CAD build for the part. Positions are in the model's coordinates, mm. A direction names the side the tool comes from. Round coordinates to 2 decimals unless told otherwise and drop trailing zeros. Use a Markdown table: item, result. Add a question column.
(1) Wall check: L1, parallel to X at y = 8.2, z = 85.5; L2, parallel to Z at x = 17.5, y = 6.5; L3, parallel to Z at x = -13, y = 11.3. Give the ranges that are in metal, low to high.
(2) Flat gauge pins, fed straight in: P1, Ø1.5, axis at x = -23.5, z = -40, coming from the -Y side; P2, Ø18.5, axis at x = -14.5, z = 74.5, coming from the +Y side; P3, Ø10, axis at x = 15, z = -91, coming from the -Y side; P4, Ø16, axis at x = -32.5, z = 37.5, coming from the -Y side. Where does each tip first touch, or does it go through?
(3) Two-plate mould, pull along X, no slides. Class faces 4 (the face through (18, 11, -54)), 5 (the face through (-65, 8, 2)), 6 (the face through (13, 0, -2)), 7 (the face through (-34.4, 5, -5.6)): released by +X, released by -X, zero draft, split by the parting line, or undercut.
(4) Band-saw the part on A-A, the plane x = -3.5. Give the number of separate pieces and of enclosed holes in the cut face, and give its area (3 significant figures).
(5) Which spindle directions (+Z, -Z, +X, -X, +Y, -Y) get a long thin tool onto all of the face, cutting with end or side? Do faces 1 (the face through (23.114, 5.93, -60.372)), 2 (the face through (-3, 13, 92.6)), 3 (the face through (27.662, 7.528, 82.922)). Say none if no direction does.
from build123d import *

# Parameters (mm, degrees)
SKETCH1_W           = 130
SKETCH1_H           = 240
BOSS_EXTRUDE1_DEPTH = 16
SKETCH7_W           = 76.2
SKETCH7_H           = 61.2
CUT_EXTRUDE5_DEPTH  = 6
SKETCH2_R           = 2.6
CUT_EXTRUDE1_DEPTH  = 11
SKETCH8_R           = 27.1
CUT_EXTRUDE6_DEPTH  = 6
SKETCH9_R           = 2.6
CUT_EXTRUDE7_DEPTH  = 11
SKETCH5_R           = 1.55
CUT_EXTRUDE3_DEPTH  = 17
SKETCH4_R           = 10
CUT_EXTRUDE2_DEPTH  = 5
SKETCH11_R          = 10
CUT_EXTRUDE8_DEPTH  = 6
FILLET1_R           = 4
CHAMFER3_SIZE       = 2
CHAMFER1_SIZE       = 1
CHAMFER2_SIZE       = 0.5


with BuildPart() as part:
    # Sketch1 → Boss-Extrude1 (new body)
    with BuildSketch(Plane(origin=(0, 0, 0), x_dir=(1, 0, 0), z_dir=(0, 1, 0))):
        Rectangle(SKETCH1_W, SKETCH1_H)
    extrude(amount=BOSS_EXTRUDE1_DEPTH)

    # Sketch7 → Cut-Extrude5 (cut)
    with BuildSketch(Plane(origin=(0, 16, 0), x_dir=(1, 0, 0), z_dir=(0, 1, 0))):
        with Locations((-3, -62)):
            Rectangle(SKETCH7_W, SKETCH7_H)
    extrude(amount=-CUT_EXTRUDE5_DEPTH, mode=Mode.SUBTRACT)

    # Sketch2 → Cut-Extrude1 (cut, through all)
    with BuildSketch(Plane(origin=(0, 10, 0), x_dir=(1, 0, 0), z_dir=(0, 1, 0))):
        with Locations((-34, -85.5)):
            Circle(SKETCH2_R)
        with Locations((-34, -38.5)):
            Circle(SKETCH2_R)
        with Locations((28, -38.5)):
            Circle(SKETCH2_R)
        with Locations((28, -85.5)):
            Circle(SKETCH2_R)
    extrude(amount=-CUT_EXTRUDE1_DEPTH, mode=Mode.SUBTRACT)

    # Sketch8 → Cut-Extrude6 (cut)
    with BuildSketch(Plane(origin=(0, 16, 0), x_dir=(1, 0, 0), z_dir=(0, 1, 0))):
        with Locations((-13, 8)):
            Circle(SKETCH8_R)
    extrude(amount=-CUT_EXTRUDE6_DEPTH, mode=Mode.SUBTRACT)

    # Sketch9 → Cut-Extrude7 (cut, through all)
    with BuildSketch(Plane(origin=(0, 10, 0), x_dir=(1, 0, 0), z_dir=(0, 1, 0))):
        with Locations((-32, 8)):
            Circle(SKETCH9_R)
        with Locations((-3.5, 24.454482672)):
            Circle(SKETCH9_R)
        with Locations((-3.5, -8.454482672)):
            Circle(SKETCH9_R)
    extrude(amount=-CUT_EXTRUDE7_DEPTH, mode=Mode.SUBTRACT)

    # Sketch5 → Cut-Extrude3 (cut, through all)
    with BuildSketch(Plane(origin=(0, 16, 0), x_dir=(1, 0, 0), z_dir=(0, 1, 0))):
        with Locations((-18.5, 51.5)):
            Circle(SKETCH5_R)
        with Locations((-18.5, 88.5)):
            Circle(SKETCH5_R)
        with Locations((18.5, 88.5)):
            Circle(SKETCH5_R)
        with Locations((18.5, 51.5)):
            Circle(SKETCH5_R)
    extrude(amount=-CUT_EXTRUDE3_DEPTH, mode=Mode.SUBTRACT)

    # Sketch4 → Cut-Extrude2 (cut)
    with BuildSketch(Plane.XZ):
        with Locations((-34, 85.5)):
            Circle(SKETCH4_R)
        with Locations((28, 85.5)):
            Circle(SKETCH4_R)
        with Locations((28, 38.5)):
            Circle(SKETCH4_R)
        with Locations((-34, 38.5)):
            Circle(SKETCH4_R)
        with Locations((-32, -8)):
            Circle(SKETCH4_R)
        with Locations((-3.5, 8.454482672)):
            Circle(SKETCH4_R)
        with Locations((-3.5, -24.454482672)):
            Circle(SKETCH4_R)
        with Locations((-18.5, -51.5)):
            Circle(SKETCH4_R)
        with Locations((-18.5, -88.5)):
            Circle(SKETCH4_R)
        with Locations((18.5, -88.5)):
            Circle(SKETCH4_R)
        with Locations((18.5, -51.5)):
            Circle(SKETCH4_R)
    extrude(amount=-CUT_EXTRUDE2_DEPTH, mode=Mode.SUBTRACT)

    # Sketch11 → Cut-Extrude8 (cut)
    with BuildSketch(Plane.XZ.offset(-5)):
        with Locations((18.5, -88.5)):
            Circle(SKETCH11_R)
        with Locations((-18.5, -88.5)):
            Circle(SKETCH11_R)
        with Locations((-18.5, -51.5)):
            Circle(SKETCH11_R)
        with Locations((18.5, -51.5)):
            Circle(SKETCH11_R)
    extrude(amount=-CUT_EXTRUDE8_DEPTH, mode=Mode.SUBTRACT)

    # Fillet1
    fillet1_edges = [part.edges().sort_by_distance(p)[0] for p in [
        (35.1, 13, 31.4),
        (35.1, 13, 92.6),
        (-41.1, 13, 92.6),
        (-41.1, 13, 31.4),
        (-65, 8, -120),
        (65, 8, -120),
        (65, 8, 120),
        (-65, 8, 120),
    ]]
    fillet(fillet1_edges, radius=FILLET1_R)

    # Chamfer3
    chamfer3_edges = [part.edges().sort_by_distance(p)[0] for p in [
        (-65, 0, 0),
        (-65, 16, 0),
        (0, 0, -120),
        (65, 0, 0),
        (0, 0, 120),
        (63.828427125, 0, 118.828427125),
        (-63.828427125, 0, 118.828427125),
        (63.828427125, 0, -118.828427125),
        (-63.828427125, 0, -118.828427125),
        (0, 16, -120),
        (0, 16, 120),
        (65, 16, 0),
        (63.828427125, 16, 118.828427125),
        (-63.828427125, 16, 118.828427125),
        (63.828427125, 16, -118.828427125),
        (-63.828427125, 16, -118.828427125),
    ]]
    chamfer(chamfer3_edges, length=CHAMFER3_SIZE)

    # Chamfer1
    chamfer1_edges = [part.edges().sort_by_distance(p)[0] for p in [
        (-13.5, 0, -24.454482672),
        (-13.5, 0, 8.454482672),
        (-42, 0, -8),
        (-44, 0, 38.5),
        (18, 0, 38.5),
        (18, 0, 85.5),
        (8.5, 0, -88.5),
        (8.5, 0, -51.5),
        (-44, 0, 85.5),
        (35.1, 16, 62),
        (-3, 16, 92.6),
        (-41.1, 16, 62),
        (-3, 16, 31.4),
        (33.928427125, 16, 32.571572875),
        (33.928427125, 16, 91.428427125),
        (-39.928427125, 16, 91.428427125),
        (-39.928427125, 16, 32.571572875),
        (-40.1, 16, -8),
        (-28.5, 0, -88.5),
        (-28.5, 0, -51.5),
    ]]
    chamfer(chamfer1_edges, length=CHAMFER1_SIZE)

    # Chamfer2
    chamfer2_edges = [part.edges().sort_by_distance(p)[0] for p in [
        (-6.1, 5, -24.454482672),
        (-6.1, 5, 8.454482672),
        (-34.6, 5, -8),
        (-36.6, 5, 38.5),
        (25.4, 5, 38.5),
        (25.4, 5, 85.5),
        (-36.6, 5, 85.5),
        (16.95, 11, -51.5),
        (-20.05, 11, -51.5),
        (-20.05, 11, -88.5),
        (16.95, 11, -88.5),
        (25.4, 10, 85.5),
        (25.4, 10, 38.5),
        (-36.6, 10, 38.5),
        (-36.6, 10, 85.5),
        (-34.6, 10, -8),
        (-6.1, 10, -24.454482672),
        (-6.1, 10, 8.454482672),
        (16.95, 16, -51.5),
        (16.95, 16, -88.5),
        (-20.05, 16, -88.5),
        (-20.05, 16, -51.5),
    ]]
    chamfer(chamfer2_edges, length=CHAMFER2_SIZE)


solid = part.part
Return value:
| question | item | result |
|---|---|---|
| 1 | L1 | -65 to -36.6, -31.4 to 25.4, 30.6 to 65 |
| 1 | L2 | -120 to -98.45, -78.55 to -61.45, -41.55 to 120 |
| 1 | L3 | -120 to -35.1, 19.1 to 31.4, 92.6 to 120 |
| 2 | P1 | y = 0 |
| 2 | P2 | y = 10 |
| 2 | P3 | y = 11 |
| 2 | P4 | y = 5 |
| 3 | face 4 | undercut |
| 3 | face 5 | released by -X |
| 3 | face 6 | zero draft |
| 3 | face 7 | undercut |
| 4 | separate pieces | 3 |
| 4 | enclosed holes | 0 |
| 4 | area | 2,900 mm^2 |
| 5 | face 1 | -Y |
| 5 | face 2 | +Y |
| 5 | face 3 | +Y, -Y |
